```python
from build123d import *

# Parameters (mm, degrees)
SKETCH1_W               = 210
SKETCH1_H               = 105
BOSS_EXTRUDE1_DEPTH     = 20
SKETCH3_W               = 18
SKETCH3_H               = 18
CUT_EXTRUDE1_DEPTH      = 5
SKETCH6_W               = 18
SKETCH6_H               = 20
BOSS_EXTRUDE2_DEPTH     = 10
SKETCH7_W               = 18
SKETCH7_H               = 7
CUT_EXTRUDE2_DEPTH      = 3
SKETCH8_W               = 18
SKETCH8_H               = 7
BOSS_EXTRUDE3_DEPTH     = 120
CUT_EXTRUDE4_DEPTH      = 261.74205403
CUT_EXTRUDE4_DEPTH_BACK = 261.74205403
SKETCH12_W              = 150
SKETCH12_H              = 25
CUT_EXTRUDE5_DEPTH      = 176.159501213
SKETCH15_W              = 30
SKETCH15_H              = 9
BOSS_EXTRUDE4_DEPTH     = 105
SKETCH16_R              = 7.5
CUT_EXTRUDE11_DEPTH     = 105
SKETCH20_W              = 20
SKETCH20_H              = 25
BOSS_EXTRUDE5_DEPTH     = 20
SKETCH21_R              = 2.375
CUT_EXTRUDE9_DEPTH      = 20
FILLET1_R               = 1
BOSS_EXTRUDE6_DEPTH     = 18
BOSS_EXTRUDE7_DEPTH     = 18
SCALE1_SCALE            = 0.4


with BuildPart() as part:
    # Sketch1 → Boss-Extrude1 (new body)
    with BuildSketch(Plane.XY):
        with Locations((4.88372093, -6.511627907)):
            Rectangle(SKETCH1_W, SKETCH1_H)
    extrude(amount=BOSS_EXTRUDE1_DEPTH)

    # Sketch3 → Cut-Extrude1 (cut)
    with BuildSketch(Plane.XY.offset(20)):
        with Locations((-91.11627907, -50.011627907)):
            Rectangle(SKETCH3_W, SKETCH3_H)
        with Locations((100.88372093, -50.011627907)):
            Rectangle(SKETCH3_W, SKETCH3_H)
    extrude(amount=-CUT_EXTRUDE1_DEPTH, mode=Mode.SUBTRACT)

    # Sketch6 → Boss-Extrude2 (add)
    with BuildSketch(Plane.XY.offset(15)):
        with Locations((-91.11627907, -51.011627907)):
            Rectangle(SKETCH6_W, SKETCH6_H)
        with Locations((100.88372093, -51.011627907)):
            Rectangle(SKETCH6_W, SKETCH6_H)
    extrude(amount=BOSS_EXTRUDE2_DEPTH)

    # Sketch7 → Cut-Extrude2 (cut)
    with BuildSketch(Plane.XY.offset(25)):
        with Locations((-91.11627907, -54.511627907)):
            Rectangle(SKETCH7_W, SKETCH7_H)
        with Locations((100.88372093, -54.511627907)):
            Rectangle(SKETCH7_W, SKETCH7_H)
    extrude(amount=-CUT_EXTRUDE2_DEPTH, mode=Mode.SUBTRACT)

    # Sketch8 → Boss-Extrude3 (add)
    with BuildSketch(Plane.XY.offset(22)):
        with Locations((-91.11627907, -54.511627907)):
            Rectangle(SKETCH8_W, SKETCH8_H)
        with Locations((100.88372093, -54.511627907)):
            Rectangle(SKETCH8_W, SKETCH8_H)
    extrude(amount=BOSS_EXTRUDE3_DEPTH)

    # Sketch9 → Cut-Extrude4 (cut, two sides: drawn at the far end of the back side and taken through both)
    with BuildSketch(Plane(origin=(109.88372093, 0, 0), x_dir=(0, 0, -1), z_dir=(1, 0, 0)).offset(-CUT_EXTRUDE4_DEPTH_BACK)):
        Polygon((-490.55895682, 10.448720548), (-142, -51.011627907), (-102.301027263, -58.011627907), (246.257929557, -119.471976362), (123.337232647, -816.589890001), (-613.479653729, -686.669193091), align=None)
    extrude(amount=CUT_EXTRUDE4_DEPTH + CUT_EXTRUDE4_DEPTH_BACK, mode=Mode.SUBTRACT)

    # Sketch12 → Cut-Extrude5 (cut, through all)
    with BuildSketch(Plane.XY.offset(20)):
        with Locations((4.88372093, 17.488372093)):
            Rectangle(SKETCH12_W, SKETCH12_H)
        with Locations((4.88372093, -30.511627907)):
            Rectangle(SKETCH12_W, SKETCH12_H)
    extrude(amount=-CUT_EXTRUDE5_DEPTH, mode=Mode.SUBTRACT)

    # Sketch15 → Boss-Extrude4 (add)
    with BuildSketch(Plane(origin=(0, 45.988372093, 0), x_dir=(1, 0, 0), z_dir=(0, 1, 0))):
        with Locations((-85.11627907, 4.5)):
            Rectangle(SKETCH15_W, SKETCH15_H)
        with Locations((94.88372093, 4.5)):
            Rectangle(SKETCH15_W, SKETCH15_H)
    extrude(amount=-BOSS_EXTRUDE4_DEPTH)

    # Sketch16 → Cut-Extrude11 (cut)
    with BuildSketch(Plane(origin=(0, 45.988372093, 0), x_dir=(1, 0, 0), z_dir=(0, 1, 0))):
        with Locations(Location((-82.99127907, -5, 0), (0, 0, 270))):
            Circle(SKETCH16_R)
        with Locations(Location((92.75872093, -5, 0), (0, 0, 270))):
            Circle(SKETCH16_R)
    extrude(amount=-CUT_EXTRUDE11_DEPTH, mode=Mode.SUBTRACT)

    # Sketch20 → Boss-Extrude5 (add)
    with BuildSketch(Plane.XY.offset(20)):
        with Locations((4.88372093, 17.488372093)):
            Rectangle(SKETCH20_W, SKETCH20_H)
    extrude(amount=-BOSS_EXTRUDE5_DEPTH)

    # Sketch21 → Cut-Extrude9 (cut)
    with BuildSketch(Plane.XY.offset(20)):
        with Locations((-0.81877907, 11.938372093)):
            Circle(SKETCH21_R)
        with Locations((10.55622093, 11.788372093)):
            Circle(SKETCH21_R)
        with Locations(Location((10.55622093, 23.188372093, 0), (0, 0, 180))):
            Circle(SKETCH21_R)
        with Locations(Location((-0.81877907, 23.038372093, 0), (0, 0, 180))):
            Circle(SKETCH21_R)
    extrude(amount=-CUT_EXTRUDE9_DEPTH, mode=Mode.SUBTRACT)

    # Fillet1
    fillet1_edges = [part.edges().sort_by_distance(p)[0] for p in [
        (-100.11627907, -6.511627907, -9),
        (-70.11627907, -6.511627907, -9),
        (109.88372093, -6.511627907, -9),
        (79.88372093, -6.511627907, -9),
    ]]
    fillet(fillet1_edges, radius=FILLET1_R)

    # Sketch23 → Boss-Extrude6 (add)
    with BuildSketch(Plane.ZY.offset(100.11627907)):
        Polygon((20, -18.461238028), (27.217256565, -51.011627907), (20, -51.011627907), align=None)
    extrude(amount=-BOSS_EXTRUDE6_DEPTH)

    # Sketch25 → Boss-Extrude7 (add)
    with BuildSketch(Plane(origin=(109.88372093, 0, 0), x_dir=(0, 0, -1), z_dir=(1, 0, 0))):
        Polygon((-20, -18.461238028), (-27.217256565, -51.011627907), (-20, -51.011627907), align=None)
    extrude(amount=-BOSS_EXTRUDE7_DEPTH)


with BuildPart() as part_1:
    # Scale1: scaled about (4.883781695, -9.980592238, 12.902521202)
    add(part.part.scale(SCALE1_SCALE).moved(Location((2.930269017, -5.988355343, 7.741512721))))


solid = part_1.part
```
Check sheet for the modelled part. Datum: model origin and axes. Units: mm. A direction names the side the tool comes from. Give positions to 0.01 mm unless a question says otherwise; leave off trailing zeros. Write each loop counter-clockwise with the first axis right and the second up, starting at its lowest first coordinate (ties: lowest second). Pieces come first, ordered by that corner, then holes. Notation, with made-up numbers: (1, -12.75) -> (57, -12.75) arc R10 cw to (57, -1.75) -> close; hole circle Ø3 at (67.5, 30). An arc over 180 degrees is marked (long way). Use CSV: the item, a comma, the result in double quotes. Start each with the question number.
Q1. Tool access check on faces 4 (the flat face through (41, -8, 4.142)), 5 (the flat face through (34.884, -9, 6)), 6 (the flat face through (4, -13.193, 12)), 7 (the flat face through (-34, -29.193, 33)), 8 (the flat face through (4, 0, 7.742)). Record the directions out of +Z, -Z, +X, -X, +Y, -Y that give a thin tool (end or side, any length) a straight path to the whole face; none if there is none.
Q2. Cross-section at B-B on x = -2.5. Enter the section's corners in (y, z), and give its area (3 significant figures).
Q3. Cross-section at A-A on z = 23.5. Enter the section's corners in (x, y), and give its area (3 significant figures).
Q4. Cross-section at C-C on y = -16.5. Enter the section's corners in (x, z), and give its area (3 significant figures).
Q5. Release check for a two-part mould opening along Y. For faces 1 (the flat face through (22, -3.993, 12)), 2 (the flat face through (-34, -30.393, 16)), 3 (the flat face through (-34, -26.393, 41)) record: +Y half, -Y half, draft (parallel to the pull), parting line (faces both ways), or undercut.
Q6. Depth check by flat-ended pin: P1, Ø10, axis at x = 14, y = -21.5, coming from the +Z side; P2, Ø4, axis at x = 3, z = 12.5, coming from the -Y side; P3, Ø2, axis at x = 7.15, y = 3.29, coming from the -Z side. Enter the tip coordinate at first touch or a pass-through.
Q7. Cross-section at D-D on z = 11. Count the separate pieces of the cut face and the enclosed holes in it, and give its area (3 significant figures).
Q8. Scan lines: line 1 along Y through (x, z) = (-11, 13); line 2 along X through (y, z) = (-10, 10); line 3 along X through (y, z) = (-16.5, 8.5). Record each from-to range of solid material in increasing order.
Working result:
1,face 4,"-Z, +X, -X, +Y, -Y"
1,face 5,"-Z"
1,face 6,"+Z, -Z"
1,face 7,"+Z, +X, -X, -Y"
1,face 8,"-Z, +Y, -Y"
2,outline,"(-29.59, 7.74) -> (-23.19, 7.74) -> (-23.19, 15.74) -> (-29.59, 15.74) -> close; (-13.19, 7.74) -> (-3.99, 7.74) -> (-3.99, 15.74) -> (-13.19, 15.74) -> close; (6.01, 7.74) -> (12.41, 7.74) -> (12.41, 15.74) -> (6.01, 15.74) -> close"
2,area,"176 mm^2"
3,outline,"(-37.12, -29.19) -> (-29.92, -29.19) -> (-29.92, -26.39) -> (-37.12, -26.39) -> close; (39.68, -29.19) -> (46.88, -29.19) -> (46.88, -26.39) -> (39.68, -26.39) -> close"
3,area,"40.3 mm^2"
4,outline,"(-37.12, 4.54) arc R0.4 ccw to (-36.72, 4.14) -> (-25.52, 4.14) arc R0.4 ccw to (-25.12, 4.54) -> (-25.12, 15.74) -> (-29.92, 15.74) -> (-29.92, 16.43) -> (-37.12, 16.43) -> close; (34.88, 4.54) arc R0.4 ccw to (35.28, 4.14) -> (46.48, 4.14) arc R0.4 ccw to (46.88, 4.54) -> (46.88, 16.43) -> (39.68, 16.43) -> (39.68, 15.74) -> (34.88, 15.74) -> close; hole circle Ø6 at (-30.27, 9.74); hole circle Ø6 at (40.03, 9.74)"
4,area,"232 mm^2"
5,face 1,"undercut"
5,face 2,"-Y half"
5,face 3,"+Y half"
6,P1,"stops at z = 15.74"
6,P2,"stops at y = -29.59"
6,P3,"stops at z = 7.74"
7,separate pieces,"3"
7,enclosed holes,"7"
7,area,"1,940 mm^2"
8,line 1,"y = -29.59 to -23.19, -13.19 to -3.99, 6.01 to 12.41"
8,line 2,"x = -37.12 to -33.26, -27.28 to 37.04, 43.02 to 46.88"
8,line 3,"x = -37.12 to -33, -27.54 to -25.12, 34.88 to 37.3, 42.76 to 46.88"
